For this review, take the finished solid that the model builds, in its own axes (mm). A direction names the side the tool comes from. Coordinates: 2 decimals unless noted, no trailing zeros. Loops run counter-clockwise (first coordinate to the right, second up) from the corner with the lowest first, then second, coordinate; pieces in that order, holes last. Notation, with made-up numbers: M 3,29 L 18,29 A13 ccw 18,47 Z; hole C -30,-17.75 d6. An arc over 180 degrees is marked long. Put each result on its own line as item: value.
```python
from build123d import *

# Parameters (mm, degrees)
SKETCH1_W                       = 40.894
SKETCH1_H                       = 25.4
REVOLVE1_ANGLE                  = 180
BOSS_EXTRUDE1_REACH             = 27.4
SKETCH3_W                       = 25.654
SKETCH3_H                       = 4.572
BOSS_EXTRUDE1_DIRECTION_2_REACH = 27.4
SKETCH4_W                       = 25.654
SKETCH4_H                       = 24.524924672
CUT_EXTRUDE1_DEPTH              = 4.572
SKETCH5_W                       = 3.81
SKETCH5_H                       = 2.032
BOSS_EXTRUDE2_DEPTH             = 25.654
SKETCH8_W                       = 6.35
SKETCH8_H                       = 30.865764514
CUT_REVOLVE2_ANGLE              = 40
CUT_REVOLVE2_OTHER_WAY_ANGLE    = 40
CUT_EXTRUDE3_DEPTH              = 45.72


with BuildPart() as part:
    # Sketch1 → Revolve1 (revolve)
    with BuildSketch(Plane(origin=(0, 0, 0), x_dir=(1, 0, 0), z_dir=(0, 1, 0))):
        with Locations((20.447, -12.7)):
            Rectangle(SKETCH1_W, SKETCH1_H)
    revolve(axis=Axis((0, 0, 0), (1, 0, 0)), revolution_arc=REVOLVE1_ANGLE)

    # Sketch2 → Cut-Revolve1 (revolve, cut)
    with BuildSketch(Plane(origin=(0, 0, 0), x_dir=(1, 0, 0), z_dir=(0, 1, 0))):
        Polygon((0, 0), (41.402, 0), (41.402, -20.701), (40.132, -20.701), (1.27, -20.701), (0, -20.701), align=None)
    revolve(axis=Axis((0, 0, 0), (1, 0, 0)), mode=Mode.SUBTRACT)

    # Sketch3 → Boss-Extrude1 (add, up to next)
    with BuildSketch(Plane.XY, mode=Mode.PRIVATE) as boss_extrude1_sk1:
        with Locations((20.447, -13.97)):
            Rectangle(SKETCH3_W, SKETCH3_H)
    boss_extrude1_tool1 = extrude(boss_extrude1_sk1.sketch, amount=BOSS_EXTRUDE1_REACH, mode=Mode.PRIVATE) - part.part
    add(boss_extrude1_tool1.solids().sort_by_distance((20.447, -13.97, 0))[0])

    # Sketch3 → Boss-Extrude1 direction 2 (add, up to next)
    with BuildSketch(Plane.XY, mode=Mode.PRIVATE) as boss_extrude1_direction_2_sk1:
        with Locations((20.447, -13.97)):
            Rectangle(SKETCH3_W, SKETCH3_H)
    boss_extrude1_direction_2_tool1 = extrude(boss_extrude1_direction_2_sk1.sketch, amount=-BOSS_EXTRUDE1_DIRECTION_2_REACH, mode=Mode.PRIVATE) - part.part
    add(boss_extrude1_direction_2_tool1.solids().sort_by_distance((20.447, -13.97, 0))[0])

    # Sketch4 → Cut-Extrude1 (cut)
    with BuildSketch(Plane(origin=(0, -11.684, 0), x_dir=(1, 0, 0), z_dir=(0, 1, 0))):
        with Locations((20.447, 0)):
            Rectangle(SKETCH4_W, SKETCH4_H)
    extrude(amount=-CUT_EXTRUDE1_DEPTH, mode=Mode.SUBTRACT)

    # Sketch5 → Boss-Extrude2 (add)
    with BuildSketch(Plane.ZY.offset(-7.62)):
        with Locations((-10.357462336, -13.97)):
            Rectangle(SKETCH5_W, SKETCH5_H)
        with Locations((10.357462336, -13.97)):
            Rectangle(SKETCH5_W, SKETCH5_H)
    extrude(amount=-BOSS_EXTRUDE2_DEPTH)

    # Sketch8 → Cut-Revolve2 (revolve, cut)
    with BuildSketch(Plane.XY):
        with Locations((19.939, -12.892882257)):
            Rectangle(SKETCH8_W, SKETCH8_H)
    revolve(axis=Axis((23.114, 2.54, 0), (-1, 0, 0)), revolution_arc=CUT_REVOLVE2_ANGLE, mode=Mode.SUBTRACT)

    # Sketch8 → Cut-Revolve2 other way (revolve, cut)
    with BuildSketch(Plane.XY):
        with Locations((19.939, -12.892882257)):
            Rectangle(SKETCH8_W, SKETCH8_H)
    revolve(axis=Axis((23.114, 2.54, 0), (1, 0, 0)), revolution_arc=CUT_REVOLVE2_OTHER_WAY_ANGLE, mode=Mode.SUBTRACT)

    # Sketch9 → Cut-Extrude3 (cut)
    with BuildSketch(Plane(origin=(40.894, 0, 0), x_dir=(0, 0, -1), z_dir=(1, 0, 0))):
        with BuildLine():
            ThreePointArc((25.019, 0), (0, -25.019), (-25.019, 0))
            Line((-25.019, 0), (-25.4, 0))
            ThreePointArc((-25.4, 0), (0, -25.4), (25.4, 0))
            Line((25.4, 0), (25.019, 0))
        make_face()
    extrude(amount=-CUT_EXTRUDE3_DEPTH, mode=Mode.SUBTRACT)


solid = part.part
```
(1) Add section D-D (y = -7.5). Write out the cut boundary in (x, z).
Determined:
outline: M 0,-23.87 L 40.89,-23.87 L 40.89,-19.29 L 0,-19.29 Z; M 0,19.29 L 40.89,19.29 L 40.89,23.87 L 0,23.87 Z
(2) Add section B-B (z = 0). Write out the cut boundary in (x, y), plus the area to 3 significant figures.
Determined:
outline: M 0,-25.02 L 16.76,-25.02 L 16.76,-20.7 L 0,-20.7 Z; M 23.11,-25.02 L 40.89,-25.02 L 40.89,-20.7 L 23.11,-20.7 Z
area: 149 mm^2
(3) Add section A-A (x = 22.5). Write out the cut boundary in (y, z).
Determined:
outline: M -18.08,-17.3 A25.02 ccw 0,-25.02 L 0,-20.7 A20.7 cw -11.68,-17.09 L -11.68,-12.26 L -12.07,-12.26 Z; M -18.08,17.3 L -12.07,12.26 L -11.68,12.26 L -11.68,17.09 A20.7 cw 0,20.7 L 0,25.02 A25.02 ccw Z
(4) Tool access review of faces 1 (the flat face through (12, -14.986, 10)), 2 (the flat face through (19.895, -15.033, 14.745)), 3 (the flat face through (20, 0, 23)), 4 (the flat face through (12, -14, -8.452)): name each direction out of +Z, -Z, +X, -X, +Y, -Y from which nothing blocks a thin tool from reaching the whole face with its end or side.
Determined:
face 1: +X, -X
face 2: -Y
face 3: +Z, -Z, +X, -X, +Y
face 4: +X, -X, +Y
(5) For pin 1 (3 mm diameter, centred on x = 13, z = 10.5, fed in from +Y); pin 2 (0.6 mm diameter, centred on x = 28, z = 12.5, fed in from -Y); pin 3 (5 mm diameter, centred on y = -12.5, z = -8, fed in from -X), all flat-tipped, find the tip position at first contact; note any pin that passes through.
Determined:
pin 1: stops at y = -12.95
pin 2: stops at y = -21.84
pin 3: stops at x = 7.62
(6) Draft analysis for pull direction Z (two halves, no side actions). For faces 5 (the cylindrical face through (25, -25, -1)), 6 (the flat face through (12, -14, 8.452)), 7 (the flat face through (40.894, -21, 2)), state which applies: +Z half, -Z half, draft (parallel to the pull), parting line (faces both ways), or undercut.
Determined:
face 5: parting line
face 6: undercut
face 7: draft
(7) Wall thickness on line 1 along X through (y, z) = (-17, -16); line 2 along X through (y, z) = (-13.5, -8.5); line 3 along Z through (x, y) = (37.5, -5): over which ranges is each line inside the solid? List them lowest first. Write a range as [from, to].
Determined:
line 1: x = [0, 16.76], [23.11, 40.89]
line 2: x = [7.62, 16.76], [23.11, 33.27]
line 3: z = [-24.51, -20.09], [20.09, 24.51]
(8) Add section C-C (x = 15). Write out the cut boundary in (y, z).
Determined:
outline: M -16.26,-12.82 A20.7 cw -16.26,12.82 L -16.26,12.26 L -14.99,12.26 L -14.99,8.45 L -12.95,8.45 L -12.95,12.26 L -11.68,12.26 L -11.68,17.09 A20.7 cw 0,20.7 L 0,25.02 A25.02 ccw 0,-25.02 L 0,-20.7 A20.7 cw -11.68,-17.09 L -11.68,-12.26 L -12.95,-12.26 L -12.95,-8.45 L -14.99,-8.45 L -14.99,-12.26 L -16.26,-12.26 Z
